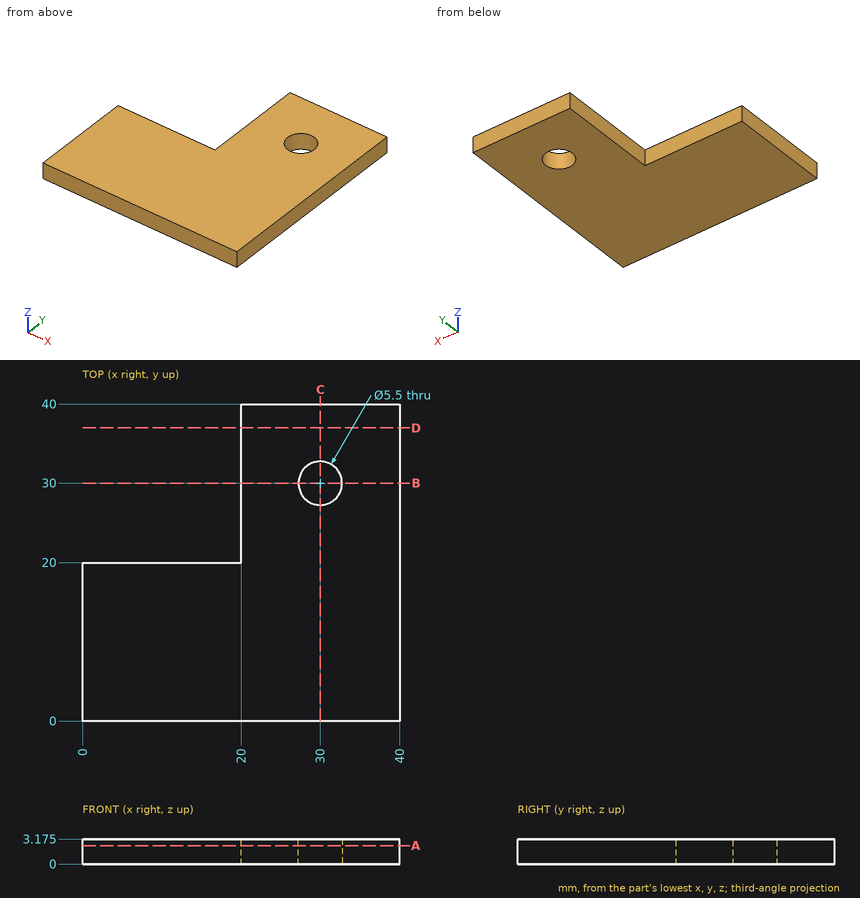
Study the drawing (mm; zero at the part's minimum x, y, z) and answer. Round coordinates to 2 decimals unless told otherwise and drop trailing zeros. Loops run counter-clockwise (first coordinate to the right, second up) from the corner with the lowest first, then second, coordinate; pieces in that order, holes last.
Q1. Section A-A, the plane z = 2.35 is taken. Determine the outline of the cut face in (x, y).
Q2. Section D-D, the plane y = 37 is taken. Determine the outline of the cut face in (x, z) (3 decimals).
Q3. Given pin 1 Ø5 at (x, y) = (30, 30) entering from -Z, flat-ended and moving along its own axis, determine where the tip first touches the part or whether it passes through.
Q4. Find the intervals of material crossed by line 1 (Y direction, x = 30, z = 1.35); line 2 (X direction, y = 36, z = 1.3); line 3 (Y direction, x = 14.5, z = 1.5), in increasing order.
Q5. Section C-C, the plane x = 30 is taken. Determine the outline of the cut face in (y, z) (3 decimals), then the cut area to 3 significant figures.
Q6. Section B-B, the plane y = 30 is taken. Determine the outline of the cut face in (x, z) (3 decimals), then the cut area to 3 significant figures.
Completed:
1. outline: (0, 0) - (40, 0) - (40, 40) - (20, 40) - (20, 20) - (0, 20) - close; hole circle Ø5.5 at (30, 30)
2. outline: (20, 0) - (40, 0) - (40, 3.175) - (20, 3.175) - close
3. pin 1: passes through
4. line 1: y = 0 to 27.25, 32.75 to 40
4. line 2: x = 20 to 40
4. line 3: y = 0 to 20
5. outline: (0, 0) - (27.25, 0) - (27.25, 3.175) - (0, 3.175) - close; (32.75, 0) - (40, 0) - (40, 3.175) - (32.75, 3.175) - close
5. area: 110 mm2
6. outline: (20, 0) - (27.25, 0) - (27.25, 3.175) - (20, 3.175) - close; (32.75, 0) - (40, 0) - (40, 3.175) - (32.75, 3.175) - close
6. area: 46.0 mm2
